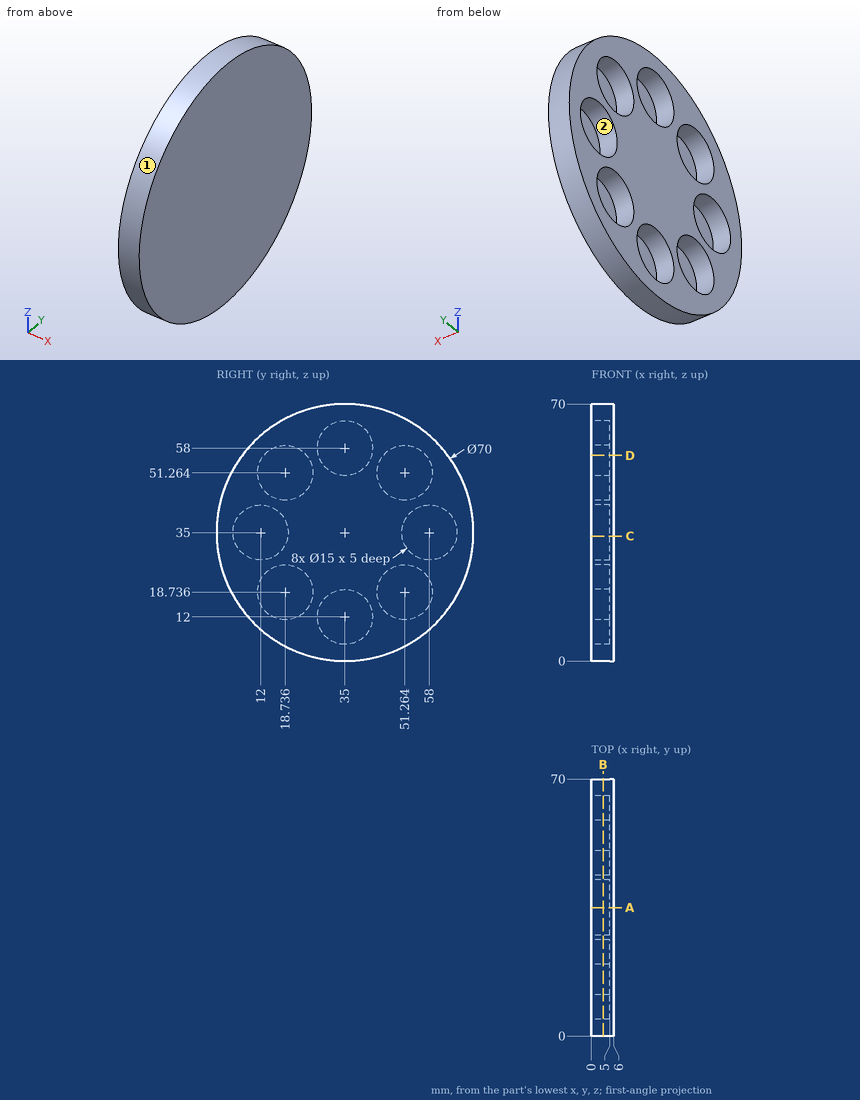
Geometry: see drawing. Coordinates: mm, zero at the bounding-box minimum. A direction names the side the tool comes from. Coordinates: 2 decimals unless noted, no trailing zeros. Order: outer loops, then holes, each group sorted by start corner. A loop starts at its lowest first (then second) coordinate and runs counter-clockwise, first axis right, second up. Notation, with made-up numbers: M -8,11 L 17,11 A29 cw 17,49 Z; hole C 50,-21.75 d7. An arc over 180 degrees is marked long. Write each question's results on one line, items separated by ' | '. Start each with the question number.
1) Section query D-D (z = 56). Return the cut outline in (x, y).
2) Contact query for flat-ended pins moving along their axis: pin 1 Ø13.5 at (y, z) = (18.74, 18.74) entering from -X; pin 2 Ø1.5 at (x, z) = (2, 39) entering from -Y; pin 3 Ø3 at (x, y) = (1, 44.5) entering from +Z. Output: stop coordinate, or through.
3) Section query A-A (y = 35). Return the cut outline in (x, z), plus the area to 3 significant figures.
4) Line query: line 1 (Z direction, x = 3.1, y = 35); line 2 (Z direction, x = 1.75, y = 37); line 3 (Z direction, x = 0.95, y = 13) (1 decimal). Output: solid intervals per line, ascending. Write a range as from..to.
5) Access query for the marked faces 1 and 2. Directions: +Z, -Z, +X, -X, +Y, -Y. A direction counts if a zero-diameter tool reaches every point of the face in a straight line with its end or side. Return the directions, or none.
6) Section query C-C (z = 34). Return the cut outline in (x, y) (1 decimal).
7) Section query B-B (x = 3.15). Give the number of separate pieces and of enclosed holes in the cut face.
Answers:
1) outline: M 0,7 L 6,7 L 6,63 L 0,63 L 0,57.08 L 5,57.08 L 5,45.45 L 0,45.45 L 0,42.23 L 5,42.23 L 5,27.77 L 0,27.77 L 0,24.55 L 5,24.55 L 5,12.92 L 0,12.92 Z
2) pin 1: stops at x = 5 | pin 2: stops at y = 0.15 | pin 3: stops at z = 69.07
3) outline: M 0,0 L 6,0 L 6,70 L 0,70 L 0,65.5 L 5,65.5 L 5,50.5 L 0,50.5 L 0,19.5 L 5,19.5 L 5,4.5 L 0,4.5 Z | area: 270 mm^2
4) line 1: z = 0..4.5, 19.5..50.5, 65.5..70 | line 2: z = 0.06..4.77, 19.23..50.77, 65.23..69.94 | line 3: z = 7.8..13.9, 23.6..27.6, 42.4..46.4, 56.1..62.2
5) face 1: +X, -X | face 2: -X
6) outline: M 0,0 L 6,0 L 6,70 L 0,70 L 0,65.4 L 5,65.4 L 5,50.6 L 0,50.6 L 0,19.4 L 5,19.4 L 5,4.6 L 0,4.6 Z
7) separate pieces: 1 | enclosed holes: 8
